For this review, take the finished solid that the model builds, in its own axes (mm). Face numbers are marked on the shaded views. A direction names the side the tool comes from. Round coordinates to 2 decimals unless told otherwise and drop trailing zeros. Order: outer loops, then holes, each group sorted by start corner. A loop starts at its lowest first (then second) coordinate and runs counter-clockwise, first axis right, second up. Notation, with made-up numbers: (49.5, 51) - (87.5, 51) arc R18 ccw to (87.5, 64) - close; hole circle Ø6 at (-30, 39). An arc over 180 degrees is marked (long way). One line per item, written item: value.
```python
from build123d import *

# Parameters (mm, degrees)
F0_W     = 4.3562594801
F0_H     = 11.6166975349
F0_H_2   = 6.6796019673
F0_W_2   = 8.1316875294
F0_H_3   = 4.0658414364
F0_H_4   = 2.6137568057
F1_DEPTH = 25.4


with BuildPart() as f1:
    # F0 (on Front) → F1 (new body)
    with BuildSketch(Plane.XZ):
        with Locations((-31.219872646, 17.5702543929)):
            Rectangle(F0_W, F0_H)
        Polygon((-33.3980023861, 11.7619056255), (-42.1105250716, 11.7619056255), (-42.1105250716, -20.7648463547), (5.517931655, -20.7648463547), (5.517931655, 11.7619056255), (-29.041742906, 11.7619056255), (-29.041742906, 9.1481488198), (-33.3980023861, 9.1481488198), align=None)
        Polygon((0, 41.6749008), (0, 37.6090556383), (8.1316875294, 37.6090556383), (8.1316875294, 33.5432142019), (0, 33.5432142019), (0, 20.474428311), (48.790127039, 20.474428311), (48.790127039, 41.6749008), align=None)
        Polygon((-18.5867156833, 37.6090556383), (-23.2333932072, 34.2531229749), (-23.2333932072, 33.5432142019), (0, 33.5432142019), (0, 37.6090556383), align=None)
        with Locations((-31.219872646, 26.718404144)):
            Rectangle(F0_W, F0_H_2)
        with Locations((4.0658437647, 35.5761349201)):
            Rectangle(F0_W_2, F0_H_3)
        Polygon((-23.2333932072, 37.6090556383), (-33.3980023861, 30.0582051277), (-29.041742906, 30.0582051277), (-23.2333932072, 34.2531229749), align=None)
        with Locations((-31.219872646, 10.4550272226)):
            Rectangle(F0_W, F0_H_4)
        Polygon((-18.5867156833, 37.6090556383), (-23.2333932072, 37.6090556383), (-23.2333932072, 34.2531229749), align=None)
    extrude(amount=F1_DEPTH)


solid = f1.part
```
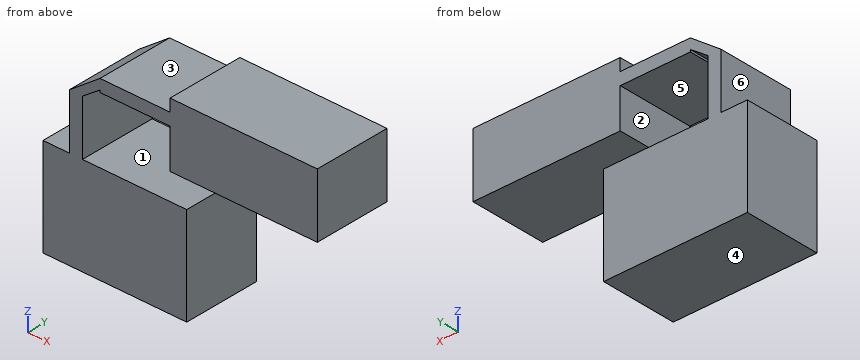
Item 1: Take a section at B-B (z = 21.5). Write out the cut boundary in (x, y), plus the area to 3 significant figures.
Returned:
outline: (-33.4, -25.4) - (-29.04, -25.4) - (-29.04, 0) - (-33.4, 0) - close; (0, -25.4) - (48.79, -25.4) - (48.79, 0) - (0, 0) - close
area: 1,350 mm^2
Item 2: Wall thickness on line 1 (X direction, y = -22.25, z = 24); line 2 (Z direction, x = -1, y = -23.5); line 3 (X direction, y = -23.75, z = -6): over which ranges is each line inside the solid? List them lowest first.
Returned:
line 1: -33.4 to -29.04, 0 to 48.79
line 2: -20.76 to 11.76, 33.54 to 37.61
line 3: -42.11 to 5.52
Item 3: Take a section at C-C (y = -19.75). Write out the cut boundary in (x, z), plus the area to 3 significant figures.
Returned:
outline: (-42.11, -20.76) - (5.52, -20.76) - (5.52, 11.76) - (-29.04, 11.76) - (-29.04, 30.06) - (-23.23, 34.25) - (-23.23, 33.54) - (0, 33.54) - (0, 20.47) - (48.79, 20.47) - (48.79, 41.67) - (0, 41.67) - (0, 37.61) - (-23.23, 37.61) - (-33.4, 30.06) - (-33.4, 11.76) - (-42.11, 11.76) - close
area: 2,780 mm^2
Item 4: Machinability: for the marked faces 1, 2 and 3, which of the approach directions +Z, -Z, +X, -X, +Y, -Y give a long, thin tool a straight path to every point of the face, cutting with its end or side? Answer none if there is none.
Returned:
face 1: +X, +Y, -Y
face 2: +Y, -Y
face 3: +Z, -X, +Y, -Y
Item 5: For P1, Ø7, axis at x = -15, y = -16, coming from the +Z side; P2, Ø1.5, axis at y = -18.5, z = 7.5, coming from the +X side; P3, Ø0.8, axis at y = -7.5, z = 34, coming from the -X side; P4, Ø3, axis at x = 1, z = 14.5, coming from the +Y side, all flat-tipped, find the tip position at first contact; note any pin that passes through.
Returned:
P1: z = 37.61
P2: x = 5.52
P3: x = -28.63
P4: through
Item 6: The part is to be moulded in two halves that separate along X. For the marked faces 4, 5 and 6, say which applies: +X half, -X half, draft (parallel to the pull), parting line (faces both ways), or undercut.
Returned:
face 4: draft
face 5: undercut
face 6: -X half
Item 7: Take a section at A-A (x = -6). Write out the cut boundary in (y, z).
Returned:
outline: (-25.4, -20.76) - (0, -20.76) - (0, 11.76) - (-25.4, 11.76) - close; (-25.4, 33.54) - (0, 33.54) - (0, 37.61) - (-25.4, 37.61) - close
Item 8: Take a section at D-D (z = -8). Write out the cut boundary in (x, y), plus the area to 3 significant figures.
Returned:
outline: (-42.11, -25.4) - (5.52, -25.4) - (5.52, 0) - (-42.11, 0) - close
area: 1,210 mm^2
